Could you check a few things on this model? Use its own coordinates, in mm. A direction names the side the tool comes from. Give positions to 0.01 mm unless a question says otherwise; leave off trailing zeros. Order: outer loops, then holes, each group sorted by start corner. A loop starts at its lowest first (then second) coordinate and runs counter-clockwise, first axis right, second up. Notation, with made-up numbers: (69, -24) -> (75, -24) arc R18 ccw to (75, -20) -> close; hole circle Ø10 at (39.5, 0.5). An arc over 180 degrees is marked (long way). Answer as CSV lines item,"result". Start each with the question number.
(1) I need wall thicknesses on L1, parallel to X at y = -7, z = -38.25; L2, parallel to Y at x = -3, z = 24.5; L3, parallel to X at y = 1.75, z = 55.5. Which ranges of each line are inside material? Lowest first, please.
(2) We'd pull the mould along Y, two halves only. Please class faces 4 (the face through (35, 0, 10)), 5 (the face through (176.9, -4.52, -37.4)), 6 (the face through (169.576, -5, -36)): released by +Y, released by -Y, zero draft, split by the parting line, or undercut.
(3) I want a section at A-A (z = 42.5). Please give me the cut outline in (x, y).
(4) Will these pins go through, and if not, where does the flat tip stop? pin 1 Ø7 at (y, z) = (-6, -37) entering from +X; pin 2 Ø10 at (x, z) = (112.5, 23.5) entering from -Y; pin 3 Ø1.5 at (y, z) = (2, 62.5) entering from -X; pin 4 Ø6 at (y, z) = (-4, 22.5) entering from +X.
(5) I want a section at B-B (x = -31.5). Please give me the cut outline in (y, z).
(6) On a 3-axis mill with a long thin cutter (end or side, diameter ignored), from which of +Z, -Z, +X, -X, +Y, -Y can I reach the whole of each face in a straight line? I mean faces 1 (the face through (183.576, -2, -34)), 2 (the face through (179.785, -6.902, -32.818)), 3 (the face through (29.576, -5, -31)). Say none if no direction works.
```python
from build123d import *

# Parameters (mm, degrees)
EXTRUDE_1_DEPTH     = 3
SKETCH_3_W          = 51.3
SKETCH_3_H          = 3
CUT_EXTRUDE_2_DEPTH = 3
SKETCH_4_W          = 4
SKETCH_4_H          = 28
SKETCH_4_W_2        = 14
SKETCH_4_H_2        = 14
EXTRUDE_2_DEPTH     = 14
CUT_EXTRUDE_3_DEPTH = 14
CUT_EXTRUDE_4_DEPTH = 14
CUT_EXTRUDE_5_DEPTH = 14
CUT_EXTRUDE_6_REACH = 216.55
SKETCH_9_R          = 2.5


with BuildPart() as part:
    # Эскиз1 → Бобышка-Вытянуть1 (new body)
    with BuildSketch(Plane(origin=(0, 0, 0), x_dir=(1, 0, 0), z_dir=(0, 1, 0))):
        Polygon((-121.424018304, 15.144551695), (-121.424018304, 41.394551695), (183.575981696, 41.394551695), (183.575981696, 15.144551695), (186.575981696, 15.144551695), (186.575981696, -11.105448305), (183.575981696, -11.105448305), (183.575981696, -37.355448305), (186.575981696, -37.355448305), (186.575981696, -63.605448305), (-118.424018304, -63.605448305), (-118.424018304, -37.355448305), (-121.424018304, -37.355448305), (-121.424018304, -11.105448305), (-118.424018304, -11.105448305), (-118.424018304, 15.144551695), align=None)
    extrude(amount=EXTRUDE_1_DEPTH)

    # Эскиз3 → Вырез-Вытянуть2 (cut)
    with BuildSketch(Plane(origin=(0, 3, 0), x_dir=(1, 0, 0), z_dir=(0, 1, 0))):
        with Locations((-95.774018304, -62.105448305)):
            Rectangle(SKETCH_3_W, SKETCH_3_H)
        with Locations((6.825981696, -62.105448305)):
            Rectangle(SKETCH_3_W, SKETCH_3_H)
        with Locations((109.425981696, -62.105448305)):
            Rectangle(SKETCH_3_W, SKETCH_3_H)
    extrude(amount=-CUT_EXTRUDE_2_DEPTH, mode=Mode.SUBTRACT)

    # Эскиз4 → Бобышка-Вытянуть2 (add)
    with BuildSketch(Plane.XZ):
        with Locations((27.575981696, -27.394551695)):
            Rectangle(SKETCH_4_W, SKETCH_4_H)
        with Locations((-111.424018304, -34.394551695)):
            Rectangle(SKETCH_4_W_2, SKETCH_4_H_2)
        with Locations((176.575981696, -34.394551695)):
            Rectangle(SKETCH_4_W_2, SKETCH_4_H_2)
        with Locations((37.575981696, -27.394551695)):
            Rectangle(SKETCH_4_W, SKETCH_4_H)
    extrude(amount=EXTRUDE_2_DEPTH)

    # Эскиз6 → Вырез-Вытянуть3 (cut)
    with BuildSketch(Plane(origin=(39.575981696, 0, 0), x_dir=(0, 0, -1), z_dir=(1, 0, 0))):
        Polygon((13.394551695, -14), (13.394551695, 0), (38.394551695, -14), align=None)
    extrude(amount=-CUT_EXTRUDE_3_DEPTH, mode=Mode.SUBTRACT)

    # Эскиз7 → Вырез-Вытянуть4 (cut)
    with BuildSketch(Plane(origin=(183.575981696, 0, 0), x_dir=(0, 0, -1), z_dir=(1, 0, 0))):
        Polygon((27.394551695, -14), (27.394551695, 0), (38.394551695, -14), align=None)
    extrude(amount=-CUT_EXTRUDE_4_DEPTH, mode=Mode.SUBTRACT)

    # Эскиз8 → Вырез-Вытянуть5 (cut)
    with BuildSketch(Plane(origin=(-104.424018304, 0, 0), x_dir=(0, 0, -1), z_dir=(1, 0, 0))):
        Polygon((27.394551695, -14), (27.394551695, 0), (38.394551695, -14), align=None)
    extrude(amount=-CUT_EXTRUDE_5_DEPTH, mode=Mode.SUBTRACT)

    # Вырез-Вытянуть6: up to this plane
    cut_extrude_6_end = Plane(origin=(169.575981696, -14, -38.394551695), z_dir=(0, 0.6178215519319037, -0.7863183388224225))
    # Эскиз9 → Вырез-Вытянуть6 (cut, up to the surface)
    with BuildSketch(Plane(origin=(0, 0, -41.394551695), x_dir=(-1, 0, 0), z_dir=(0, 0, -1)), mode=Mode.PRIVATE) as cut_extrude_6_sk1:
        with Locations((-176.575981696, -7)):
            Circle(SKETCH_9_R)
    cut_extrude_6_tool1 = split(extrude(cut_extrude_6_sk1.sketch, amount=-CUT_EXTRUDE_6_REACH, mode=Mode.PRIVATE), bisect_by=cut_extrude_6_end, keep=Keep.BOTH, mode=Mode.PRIVATE)
    add(cut_extrude_6_tool1.solids().sort_by_distance((176.575982, -7, -41.394552))[0], mode=Mode.SUBTRACT)
    # Эскиз9 → Вырез-Вытянуть6 (cut, up to the surface)
    with BuildSketch(Plane(origin=(0, 0, -41.394551695), x_dir=(-1, 0, 0), z_dir=(0, 0, -1)), mode=Mode.PRIVATE) as cut_extrude_6_sk2:
        with Locations((111.424018304, -7)):
            Circle(SKETCH_9_R)
    cut_extrude_6_tool2 = split(extrude(cut_extrude_6_sk2.sketch, amount=-CUT_EXTRUDE_6_REACH, mode=Mode.PRIVATE), bisect_by=cut_extrude_6_end, keep=Keep.BOTH, mode=Mode.PRIVATE)
    add(cut_extrude_6_tool2.solids().sort_by_distance((-111.424018, -7, -41.394552))[0], mode=Mode.SUBTRACT)


solid = part.part
```
Final values:
1,L1,"-118.42 to -113.92, -108.92 to -104.42, 25.58 to 29.58, 35.58 to 39.58, 169.58 to 174.08, 179.08 to 183.58"
1,L2,"0 to 3"
1,L3,"-118.42 to 186.58"
2,face 4,"released by -Y"
2,face 5,"undercut"
2,face 6,"zero draft"
3,outline,"(-118.42, 0) -> (186.58, 0) -> (186.58, 3) -> (-118.42, 3) -> close"
4,pin 1,"x = 183.58"
4,pin 2,"y = 0"
4,pin 3,"x = -70.12"
4,pin 4,"through"
5,outline,"(0, -41.39) -> (3, -41.39) -> (3, 63.61) -> (0, 63.61) -> close"
6,face 1,"-Z, +X, +Y, -Y"
6,face 2,"+Z, +X, -Y"
6,face 3,"+Z, -Z, -Y"
